Source: CAD feature listing. Evaluate the final solid. Frame: model axes, mm. A direction names the side the tool comes from. Round coordinates to 2 decimals unless told otherwise and drop trailing zeros. Loops run counter-clockwise (first coordinate to the right, second up) from the corner with the lowest first, then second, coordinate; pieces in that order, holes last.
Item 1: Section query A-A on y = -22.5. Return loops of the section in (x, z) (3 decimals), then the cut area to 3 significant figures.
Item 2: Ray query, L1, parallel to X at y = -29.5, z = 25; L2, parallel to X at y = -24, z = 6.35 (3 decimals); L3, parallel to Z at x = 44, y = -9. Return the intervals inside material, ascending.
Item 3: Section query C-C on z = 34.29. Return loops of the section in (x, y) (3 decimals).
Item 4: Section query D-D on y = -10. Return loops of the section in (x, z) (3 decimals).
Item 5: First-contact query: P1, Ø4, axis at x = 6.35, z = 6.35, coming from the +Y side. Flat tip, straight axial feed; report the tip coordinate or a pass-through.
Item 6: Access query for faces 1 (the flat face through (25, 0, 20)), 2 (the flat face through (12.7, -26, 20)). Directions: +Z, -Z, +X, -X, +Y, -Y. A direction counts if a zero-diameter tool reaches every point of the face in a straight line with its end or side. Return the directions, or none.
Item 7: Pull-direction query (X, two-part tool) for faces 3 (the flat face through (20.1, -8.6, 40.64)), 4 (the flat face through (38.1, -26, 20)), 5 (the flat face through (50.8, -16, 20)); classes: released by +X, released by -X, zero draft, split by the parting line, or undercut.
Item 8: Section query B-B on x = 6.35. Return loops of the section in (y, z) (3 decimals).
```python
from build123d import *

# Parameters (mm, degrees)
BOSS_EXTRUDE1_DEPTH = 40.64
SKETCH2_R           = 3.175
CUT_EXTRUDE1_DEPTH  = 73.39


with BuildPart() as part:
    # Sketch1 → Boss-Extrude1 (new body)
    with BuildSketch(Plane.XY):
        with BuildLine():
            Line((0, 0), (50.8, 0))
            Line((50.8, 0), (50.8, -31.75))
            Line((50.8, -31.75), (38.1, -31.75))
            Line((38.1, -31.75), (38.1, -20.32))
            ThreePointArc((38.1, -20.32), (25.4, -7.62), (12.7, -20.32))
            Line((12.7, -20.32), (12.7, -31.75))
            Line((12.7, -31.75), (0, -31.75))
            Line((0, -31.75), (0, 0))
        make_face()
    extrude(amount=BOSS_EXTRUDE1_DEPTH)

    # Sketch2 → Cut-Extrude1 (cut, through all)
    with BuildSketch(Plane(origin=(0, 0, 0), x_dir=(1, 0, 0), z_dir=(0, 1, 0))):
        with Locations(Location((6.35, -6.35, 0), (0, 0, 270))):
            Circle(SKETCH2_R)
        with Locations(Location((44.45, -6.35, 0), (0, 0, 90))):
            Circle(SKETCH2_R)
        with Locations(Location((6.35, -34.29, 0), (0, 0, 90))):
            Circle(SKETCH2_R)
        with Locations(Location((44.45, -34.29, 0), (0, 0, 270))):
            Circle(SKETCH2_R)
    extrude(amount=-CUT_EXTRUDE1_DEPTH, mode=Mode.SUBTRACT)


solid = part.part
```
Data:
1. outline: (0, 0) - (12.7, 0) - (12.7, 40.64) - (0, 40.64) - close; (38.1, 0) - (50.8, 0) - (50.8, 40.64) - (38.1, 40.64) - close; hole circle Ø6.35 at (6.35, 6.35); hole circle Ø6.35 at (6.35, 34.29); hole circle Ø6.35 at (44.45, 6.35); hole circle Ø6.35 at (44.45, 34.29)
1. area: 906 mm2
2. L1: x = 0 to 12.7, 38.1 to 50.8
2. L2: x = 0 to 3.175, 9.525 to 12.7, 38.1 to 41.275, 47.625 to 50.8
2. L3: z = 0 to 3.21, 9.49 to 31.15, 37.43 to 40.64
3. outline: (0, -31.75) - (3.175, -31.75) - (3.175, 0) - (0, 0) - close; (9.525, -31.75) - (12.7, -31.75) - (12.7, -20.32) arc R12.7 cw to (38.1, -20.32) - (38.1, -31.75) - (41.275, -31.75) - (41.275, 0) - (9.525, 0) - close; (47.625, -31.75) - (50.8, -31.75) - (50.8, 0) - (47.625, 0) - close
4. outline: (0, 0) - (17.998, 0) - (17.998, 40.64) - (0, 40.64) - close; (32.802, 0) - (50.8, 0) - (50.8, 40.64) - (32.802, 40.64) - close; hole circle Ø6.35 at (6.35, 6.35); hole circle Ø6.35 at (6.35, 34.29); hole circle Ø6.35 at (44.45, 6.35); hole circle Ø6.35 at (44.45, 34.29)
5. P1: passes through
6. face 1: +Z, -Z, +X, -X, +Y
6. face 2: +Z, -Z, -Y
7. face 3: zero draft
7. face 4: undercut
7. face 5: released by +X
8. outline: (-31.75, 0) - (0, 0) - (0, 3.175) - (-31.75, 3.175) - close; (-31.75, 9.525) - (0, 9.525) - (0, 31.115) - (-31.75, 31.115) - close; (-31.75, 37.465) - (0, 37.465) - (0, 40.64) - (-31.75, 40.64) - close
